Here's how the part is built. I have some questions about the finished solid (model axes, mm). A direction names the side the tool comes from. Give positions to 0.01 mm unless a question says otherwise; leave off trailing zeros. Loops run counter-clockwise (first coordinate to the right, second up) from the corner with the lowest first, then second, coordinate; pieces in that order, holes last. Notation, with made-up numbers: (76.5, 28) -> (130.5, 28) arc R24 cw to (130.5, 57) -> close; hole circle Ø8 at (32.5, -28.75). An arc over 180 degrees is marked (long way). Answer in a Markdown table with one row per item. Add a question column.
Item 1: If I drill on line 1 (X direction, y = 3.5, z = -14); line 2 (X direction, y = -3.75, z = 49); line 3 (Y direction, x = 7, z = 48), over which ranges is the centre line in solid material (lowest first)?
Item 2: We'd pull the mould along Z, two halves only. Please class faces 4 (the face through (0, -2, 76.2)), 5 (the face through (-2.451, -2.576, 71.994)), 6 (the face through (12.573, -1, -1)): released by +Z, released by -Z, zero draft, split by the parting line, or undercut.
Item 3: For P1, Ø7.5, axis at x = -1.5, z = 15, coming from the +Y side, with a flat end and sliding along its axis, tell me the tip position at first contact or that it passes through.
Item 4: If we section it at B-B (x = -2): Write out the boundary of the cut face in (y, z).
Item 5: If we section it at A-A (z = -18.5): Write out the boundary of the cut face in (x, y).
Item 6: Which directions (+Z, -Z, +X, -X, +Y, -Y) give clear straight access to the entire face, cutting with the end or side of a thin tool? Please do faces 1 (the face through (-6, -5.08, 1)), 2 (the face through (2.398, -2.576, -72.047)), 3 (the face through (-5, 0, 1)).
```python
from build123d import *

# Parameters (mm, degrees)
F0_W     = 14.986
F0_H     = 152.4
F0_W_2   = 6.858
F0_H_2   = 146.05
F0_W_3   = 5.08
F1_DEPTH = 5.08
F2_R     = 3.42899
F3_DEPTH = 3.81


# Not quite as in the source:
# - a fillet or chamfer is up to 0.001 mm smaller than in the source, because OpenCascade refuses the exact size


with BuildPart() as f1:
    # F0 (on Front) → F1 (new body)
    with BuildSketch(Plane.XZ):
        Rectangle(F0_W, F0_H)
        Rectangle(F0_W_2, F0_H_2, mode=Mode.SUBTRACT)
        with Locations((-10.033, 0)):
            Rectangle(F0_W_3, F0_H)
        with Locations((10.033, 0)):
            Rectangle(F0_W_3, F0_H)
    extrude(amount=F1_DEPTH)

    # F2 (radius 3.429 in the source; OpenCascade refuses exactly that, so slightly less here)
    f2_edges = [f1.edges().sort_by_distance(p)[0] for p in [
        (3.429, -2.54, 73.025),
        (-3.429, -2.54, 73.025),
        (-3.429, -2.54, -73.025),
        (3.429, -2.54, -73.025),
    ]]
    fillet(f2_edges, radius=F2_R)

    # F0 (on Front) → F3 (join)
    with BuildSketch(Plane.XZ):
        with Locations((10.033, 0)):
            Rectangle(F0_W_3, F0_H)
        with Locations((-10.033, 0)):
            Rectangle(F0_W_3, F0_H)
    extrude(amount=-F3_DEPTH)


solid = f1.part
```
Recorded:
| question | item | result |
|---|---|---|
| 1 | line 1 | x = -12.57 to -7.49, 7.49 to 12.57 |
| 1 | line 2 | x = -12.57 to -3.43, 3.43 to 12.57 |
| 1 | line 3 | y = -5.08 to 0 |
| 2 | face 4 | released by +Z |
| 2 | face 5 | undercut |
| 2 | face 6 | zero draft |
| 3 | P1 | stops at y = 0 |
| 4 | outline | (-5.08, -76.2) -> (0, -76.2) -> (0, -72.38) -> (-5.08, -72.38) -> close; (-5.08, 72.38) -> (0, 72.38) -> (0, 76.2) -> (-5.08, 76.2) -> close |
| 5 | outline | (-12.57, -5.08) -> (-3.43, -5.08) -> (-3.43, 0) -> (-7.49, 0) -> (-7.49, 3.81) -> (-12.57, 3.81) -> close; (3.43, -5.08) -> (12.57, -5.08) -> (12.57, 3.81) -> (7.49, 3.81) -> (7.49, 0) -> (3.43, 0) -> close |
| 6 | face 1 | +Z, -Z, +X, -X, -Y |
| 6 | face 2 | +Y, -Y |
| 6 | face 3 | +Z, -Z, +Y |
